Here's how the part is built. I have some questions about the finished solid (model axes, mm). A direction names the side the tool comes from. Round coordinates to 2 decimals unless told otherwise and drop trailing zeros. Loops run counter-clockwise (first coordinate to the right, second up) from the corner with the lowest first, then second, coordinate; pieces in that order, holes last. Notation, with made-up numbers: M 62,46.5 L 113,46.5 A30 cw 113,68.5 Z; hole C 64.5,12.25 d4. An arc over 180 degrees is marked long. Use a Markdown table: item, result.
Autodesk Inventor part; units mm, degrees
ref_plane "YZ Plane" through (0, 0, 0) normal (1, 0, 0) x (0, 1, 0)
ref_plane "XZ Plane" through (0, 0, 0) normal (0, 1, 0) x (-1, 0, 0)
ref_plane "XY Plane" through (0, 0, 0) normal (0, 0, 1) x (1, 0, 0)
sketch "スケッチ1" plane through (0, 0, 0) normal (0, 1, 0) x (-1, 0, 0)
  line L0 (0, 0) -> (30, 0)
  line L1 (30, 0) -> (30, 15)
  line L2 (30, 15) -> (0, 15)
  line L3 (0, 15) -> (0, 0)
  dimension "d0" = 30
  dimension "d1" = 15
extrude "押し出し1" add sketch "スケッチ1" along normal blind 10
sketch "スケッチ2" plane through (0, 0, 0) normal (1, 0, 0) x (0, 1, 0)
  line L0 (3, 5) -> (10, 5)
  line L1 (10, 5) -> (10, 10)
  line L2 (10, 10) -> (3, 10)
  line L3 (3, 10) -> (3, 5)
  point P0 (0, 0)
  dimension "d4" = 7
  dimension "d5" = 5
  dimension "d6" = 10
  dimension "d7" = 10
extrude "押し出し2" cut sketch "スケッチ2" against normal blind 30
hole "穴1" at (-23.0862, 0, 12.3913) direction (0, 1, 0) diameter 3 depth 10 tip angle 118 counterbore diameter 4.5 counterbore depth 2
hole "穴2" at (-7.9763, 0, 12.4901) direction (0, 1, 0) diameter 3 depth 10 tip angle 118 counterbore diameter 4.5 counterbore depth 2
hole "穴3" at (-23.2858, 0, 2.6671) direction (0, 1, 0) diameter 3 depth 10 tip angle 118 counterbore diameter 4.5 counterbore depth 2
hole "穴4" at (-8.1857, 0, 2.7752) direction (0, 1, 0) diameter 3 depth 10 tip angle 118 counterbore diameter 4.5 counterbore depth 2
properties part number "braket1"
Q1. Imagine slicing it at C-C, the plane x = -22.5. Please give me the cut outline in (y, z), then the cut area to 3 significant figures.
Return value:
| item | result |
|---|---|
| outline | M 0,0 L 10,0 L 10,1.39 L 2,1.39 L 2,0.56 L 0,0.56 Z; M 0,4.78 L 2,4.78 L 2,3.94 L 10,3.94 L 10,5 L 3,5 L 3,10 L 10,10 L 10,11.01 L 2,11.01 L 2,10.22 L 0,10.22 Z; M 0,14.56 L 2,14.56 L 2,13.77 L 10,13.77 L 10,15 L 0,15 Z |
| area | 55.3 mm^2 |
Q2. Imagine slicing it at A-A, the plane y = 8. Please give me the cut outline in (x, z), then the cut area to 3 significant figures.
Return value:
| item | result |
|---|---|
| outline | M -30,0 L 0,0 L 0,5 L -30,5 Z; M -30,10 L 0,10 L 0,15 L -30,15 Z; hole C -23.29,2.67 d3; hole C -23.09,12.39 d3; hole C -8.19,2.78 d3; hole C -7.98,12.49 d3 |
| area | 272 mm^2 |
Q3. Imagine slicing it at D-D, the plane y = 2.5. Please give me the cut outline in (x, z).
Return value:
| item | result |
|---|---|
| outline | M -30,0 L 0,0 L 0,15 L -30,15 Z; hole C -23.29,2.67 d3; hole C -23.09,12.39 d3; hole C -8.19,2.78 d3; hole C -7.98,12.49 d3 |
Q4. Will this pin go through, and if not, where does the flat tip stop? P1, Ø4, axis at x = -8.19, z = 2.78, coming from the -Y side.
Return value:
| item | result |
|---|---|
| P1 | stops at y = 2 |
Q5. For faces 4 (the flat face through (-24, 2, 11)), 5 (the cylindrical face through (-21.622, 6.056, 12.716)), which set-ups out of +Z, -Z, +X, -X, +Y, -Y let a thin tool reach every point of the face, with its end or its side?
Return value:
| item | result |
|---|---|
| face 4 | -Y |
| face 5 | +Y, -Y |
Q6. I need wall thicknesses on line 1 (Z direction, x = -11, y = 5.5); line 2 (X direction, y = 8.25, z = 12.25); line 3 (X direction, y = 4, z = 2.25). Which ranges of each line are inside material? Lowest first, please. Write a range as from..to.
Return value:
| item | result |
|---|---|
| line 1 | z = 0..5, 10..15 |
| line 2 | x = -30..-24.58, -21.59..-9.46, -6.5..0 |
| line 3 | x = -30..-24.73, -21.84..-9.59, -6.78..0 |
Q7. Imagine slicing it at B-B, the plane z = 2.25. Please give me the cut outline in (x, y).
Return value:
| item | result |
|---|---|
| outline | M -30,0 L -25.5,0 L -25.5,2 L -24.73,2 L -24.73,10 L -30,10 Z; M -21.84,2 L -21.07,2 L -21.07,0 L -10.37,0 L -10.37,2 L -9.59,2 L -9.59,10 L -21.84,10 Z; M -6.78,2 L -6,2 L -6,0 L 0,0 L 0,10 L -6.78,10 Z |
Q8. We'd pull the mould along Z, two halves only. Please class faces 1 (the flat face through (-15, 6, 5)), 2 (the flat face through (-15, 0, 8)), 3 (the flat face through (-15, 5, 15)): pulls with the +Z half, pulls with the -Z half, needs draft (parallel to the pull), parting line crosses it, or undercut.
Return value:
| item | result |
|---|---|
| face 1 | undercut |
| face 2 | needs draft |
| face 3 | pulls with the +Z half |
